from build123d import *

# Parameters (mm, degrees)
F1_DEPTH = 5.5
F2_R     = 1.45
F3_DEPTH = 25
F4_R     = 1.45
F5_DEPTH = 25


with BuildPart() as f1:
    # F0 (on Front) → F1 (new body)
    with BuildSketch(Plane.XZ):
        with BuildLine():
            ThreePointArc((-5.15, 0), (0, 5.15), (5.15, 0))
            Line((5.15, 0), (6.15, 0))
            Line((6.15, 0), (10.362235, -4.212235))
            Line((10.362235, -4.212235), (12.483555, -2.090915))
            Line((12.483555, -2.090915), (3.280338, 7.112302))
            Line((3.280338, 7.112302), (-3.280338, 7.112302))
            Line((-3.280338, 7.112302), (-12.483555, -2.090915))
            Line((-12.483555, -2.090915), (-10.362235, -4.212235))
            Line((-10.362235, -4.212235), (-6.15, 0))
            Line((-6.15, 0), (-5.15, 0))
        make_face()
    extrude(amount=F1_DEPTH)

    # F2 (on face) → F3 (cut)
    with BuildSketch(Plane(origin=(-5.19632, 0, 5.19632), x_dir=(0, -1, 0), z_dir=(-0.707107, 0, 0.707107))):
        with Locations((2.75, -7.327207)):
            Circle(F2_R)
    extrude(amount=-F3_DEPTH, mode=Mode.SUBTRACT)

    # F4 (on face) → F5 (cut)
    with BuildSketch(Plane(origin=(5.19632, 0, 5.19632), x_dir=(0, 1, 0), z_dir=(0.707107, 0, 0.707107))):
        with Locations((-2.75, -7.327207)):
            Circle(F4_R)
    extrude(amount=-F5_DEPTH, mode=Mode.SUBTRACT)


solid = f1.part
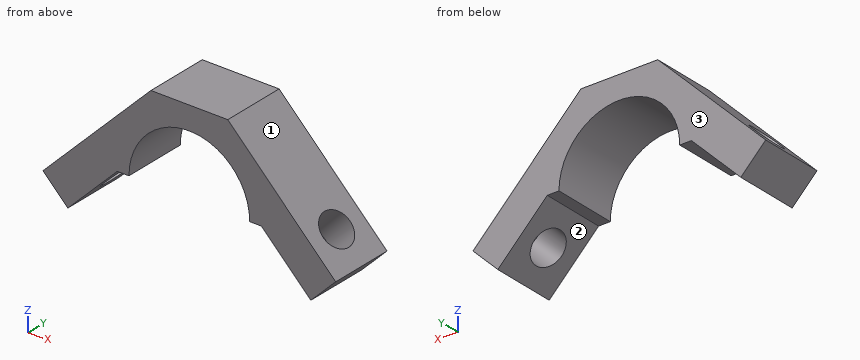
The model under review builds one solid part; all positions refer to its coordinate system, in mm. Face numbers are marked on the shaded views. Coordinates: 2 decimals unless noted, no trailing zeros. Order: outer loops, then holes, each group sorted by start corner. A loop starts at its lowest first (then second) coordinate and runs counter-clockwise, first axis right, second up. Notation, with made-up numbers: (27, 65) -> (81, 65) arc R33 ccw to (81, 101) -> close; hole circle Ø1 at (-22.75, 76). An arc over 180 degrees is marked (long way). Answer in a Markdown table with one row per item.
(1) The part is to be moulded in two halves that separate along X. For the marked faces 1, 2 and 3, say which applies: +X half, -X half, draft (parallel to the pull), parting line (faces both ways), or undercut.
Answers:
| item | result |
|---|---|
| face 1 | +X half |
| face 2 | undercut |
| face 3 | draft |
(2) Consider section C-C (x = 0). Write out the cut boundary in (y, z), plus the area to 3 significant figures.
Answers:
| item | result |
|---|---|
| outline | (-5.5, 5.15) -> (0, 5.15) -> (0, 7.11) -> (-5.5, 7.11) -> close |
| area | 10.8 mm² |
(3) Consider section A-A (y = -2). Write out the cut boundary in (x, z).
Answers:
| item | result |
|---|---|
| outline | (-12.48, -2.09) -> (-10.36, -4.21) -> (-9.13, -2.98) -> (-11.25, -0.86) -> close; (-9.5, 0.89) -> (-7.38, -1.23) -> (-6.15, 0) -> (-5.15, 0) arc R5.15 cw to (5.15, 0) -> (6.15, 0) -> (7.38, -1.23) -> (9.5, 0.89) -> (3.28, 7.11) -> (-3.28, 7.11) -> close; (9.13, -2.98) -> (10.36, -4.21) -> (12.48, -2.09) -> (11.25, -0.86) -> close |
(4) Consider section B-B (y = -0.7). Write out the cut boundary in (x, z), plus the area to 3 significant figures.
Answers:
| item | result |
|---|---|
| outline | (-12.48, -2.09) -> (-10.36, -4.21) -> (-6.15, 0) -> (-5.15, 0) arc R5.15 cw to (5.15, 0) -> (6.15, 0) -> (10.36, -4.21) -> (12.48, -2.09) -> (3.28, 7.11) -> (-3.28, 7.11) -> close |
| area | 82.3 mm² |
(5) Consider section D-D (y = -3.2). Write out the cut boundary in (x, z).
Answers:
| item | result |
|---|---|
| outline | (-12.48, -2.09) -> (-10.36, -4.21) -> (-9.23, -3.08) -> (-11.35, -0.96) -> close; (-9.4, 0.99) -> (-7.28, -1.13) -> (-6.15, 0) -> (-5.15, 0) arc R5.15 cw to (5.15, 0) -> (6.15, 0) -> (7.28, -1.13) -> (9.4, 0.99) -> (3.28, 7.11) -> (-3.28, 7.11) -> close; (9.23, -3.08) -> (10.36, -4.21) -> (12.48, -2.09) -> (11.35, -0.96) -> close |
(6) Insertion check: pin 1 (1.5 mm diameter, centred on x = -4, y = -2.5, fed in from +Z); pin 2 (0.5 mm diameter, centred on x = 5.5, y = -1.5, fed in from -Z); pin 3 (1.5 mm diameter, centred on x = -6.5, y = -1, fed in from -Z); pin 4 (1.5 mm diameter, centred on y = -4.5, z = 4, fed in from -X). Each pin has a flat end and moves straight along its axis. Give the tip position at first contact, or say it passes through.
Answers:
| item | result |
|---|---|
| pin 1 | z = 7.11 |
| pin 2 | z = 0 |
| pin 3 | z = -1.1 |
| pin 4 | x = -7.14 |
(7) Wall thickness on line 1 along X through (y, z) = (-1.7, -1.25); line 2 along X through (y, z) = (-0.35, -1); line 3 along X through (y, z) = (-3.95, 1.75): over which ranges is each line inside the solid? List them lowest first.
Answers:
| item | result |
|---|---|
| line 1 | -11.64 to -10.53, -7.7 to -7.4, 7.4 to 7.7, 10.53 to 11.64 |
| line 2 | -11.39 to -7.15, 7.15 to 11.39 |
| line 3 | -8.64 to -4.84, 4.84 to 8.64 |
